Answer from the drawing. Dimensions are ordinates in mm from the lowest x, y and z of the part. Coordinates: 2 decimals unless noted, no trailing zeros. Order: outer loops, then holes, each group sorted by start corner. A loop starts at its lowest first (then second) coordinate and runs counter-clockwise, first axis right, second up. Notation, with made-up numbers: M 55,43.25 L 98,43.25 A20 cw 98,79.25 Z; hole C 47,66 d6. An arc over 180 degrees is marked long. Use a Markdown table: item, result.
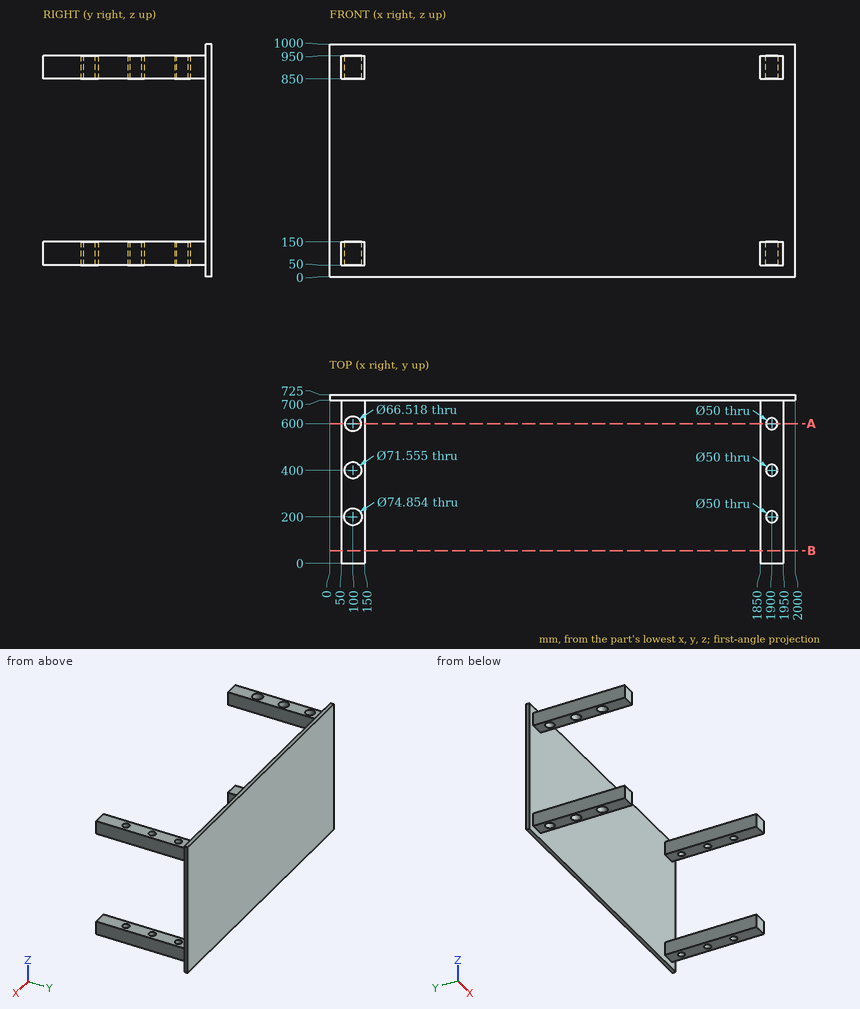
(1) A cutting plane is placed at A-A (y = 600). Give the number of separate pieces and of enclosed holes in the cut face, then the cut area to 3 significant figures.
Conclusion:
| item | result |
|---|---|
| separate pieces | 8 |
| enclosed holes | 0 |
| area | 16,700 mm2 |
(2) Given P1, Ø2, axis at x = 646, z = 788.5, coming from the -Y side, flat-ended and moving along its own axis, determine where the tip first touches the part or whether it passes through.
Conclusion:
| item | result |
|---|---|
| P1 | y = 700 |
(3) A cutting plane is placed at B-B (y = 55). Determine the outline of the cut face in (x, z).
Conclusion:
| item | result |
|---|---|
| outline | M 50,50 L 150,50 L 150,150 L 50,150 Z; M 50,850 L 150,850 L 150,950 L 50,950 Z; M 1850,50 L 1950,50 L 1950,150 L 1850,150 Z; M 1850,850 L 1950,850 L 1950,950 L 1850,950 Z |
(4) Straight lines are drawn through the part: L1, parallel to Y at x = 1900, z = 86.5; L2, parallel to Y at x = 100, z = 880; L3, parallel to X at y = 38, z = 945. For each, find the intervals that lie inside material, in ascending order.
Conclusion:
| item | result |
|---|---|
| L1 | 0 to 175, 225 to 375, 425 to 575, 625 to 725 |
| L2 | 0 to 162.57, 237.43 to 364.22, 435.78 to 566.74, 633.26 to 725 |
| L3 | 50 to 150, 1850 to 1950 |
